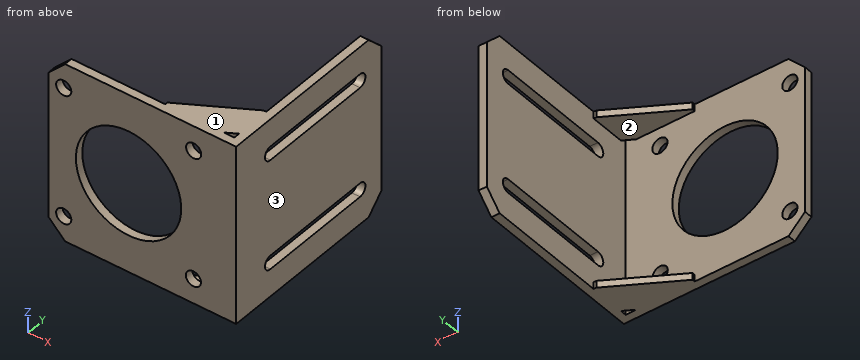
from build123d import *

# Parameters (mm, degrees)
SKETCH1_W           = 68
SKETCH1_H           = 65
BOSS_EXTRUDE1_DEPTH = 3
SKETCH2_W           = 3
SKETCH2_H           = 68
BOSS_EXTRUDE2_DEPTH = 65
CHAMFER1_SIZE       = 6
SKETCH4_R           = 2.75
SKETCH4_R_2         = 19.1
CUT_EXTRUDE2_DEPTH  = 65
CUT_EXTRUDE3_DEPTH  = 65
BOSS_EXTRUDE3_DEPTH = 2.5
BOSS_EXTRUDE4_DEPTH = 2.5


with BuildPart() as part:
    # Sketch1 → Boss-Extrude1 (new body)
    with BuildSketch(Plane(origin=(0, 0, 0), x_dir=(1, 0, 0), z_dir=(0, 1, 0))):
        Rectangle(SKETCH1_W, SKETCH1_H)
    extrude(amount=BOSS_EXTRUDE1_DEPTH)

    # Sketch2 → Boss-Extrude2 (add)
    with BuildSketch(Plane.XY.offset(32.5)):
        with Locations((32.5, 34)):
            Rectangle(SKETCH2_W, SKETCH2_H)
    extrude(amount=-BOSS_EXTRUDE2_DEPTH)

    # Chamfer1
    chamfer1_edges = [part.edges().sort_by_distance(p)[0] for p in [
        (32.5, 68, -32.5),
        (32.5, 68, 32.5),
        (-34, 1.5, -32.5),
        (-34, 1.5, 32.5),
    ]]
    chamfer(chamfer1_edges, length=CHAMFER1_SIZE)

    # Sketch4 → Cut-Extrude2 (cut)
    with BuildSketch(Plane(origin=(0, 3, 0), x_dir=(1, 0, 0), z_dir=(0, 1, 0))):
        with Locations(Location((-28.5, 23.5, 0), (0, 0, 270))):
            Circle(SKETCH4_R)
        with Locations(Location((-28.5, -23.5, 0), (0, 0, 270))):
            Circle(SKETCH4_R)
        with Locations(Location((18.6, -23.5, 0), (0, 0, 270))):
            Circle(SKETCH4_R)
        with Locations(Location((18.5, 23.5, 0), (0, 0, 270))):
            Circle(SKETCH4_R)
        with Locations(Location((-5, 0, 0), (0, 0, 270))):
            Circle(SKETCH4_R_2)
    extrude(amount=-CUT_EXTRUDE2_DEPTH, mode=Mode.SUBTRACT)

    # Sketch5 → Cut-Extrude3 (cut)
    with BuildSketch(Plane.ZY.offset(-31)):
        with BuildLine():
            Line((-17.5, 58), (-17.5, 16))
            ThreePointArc((-17.5, 16), (-20, 13.5), (-22.5, 16))
            Line((-22.5, 16), (-22.5, 58))
            ThreePointArc((-22.5, 58), (-20, 60.5), (-17.5, 58))
        make_face()
        with BuildLine():
            Line((22.5, 58), (22.5, 16))
            ThreePointArc((22.5, 16), (20, 13.5), (17.5, 16))
            Line((17.5, 16), (17.5, 58))
            ThreePointArc((17.5, 58), (20, 60.5), (22.5, 58))
        make_face()
    extrude(amount=-CUT_EXTRUDE3_DEPTH, mode=Mode.SUBTRACT)

    # Sketch6 → Boss-Extrude3 (add)
    with BuildSketch(Plane.XY.offset(32.5)):
        Polygon((6, 3), (6, 4), (30, 18), (31, 18), (31, 5.233358358), (27.171385671, 3), align=None)
    extrude(amount=-BOSS_EXTRUDE3_DEPTH)

    # Sketch7 → Boss-Extrude4 (add)
    with BuildSketch(Plane(origin=(0, 0, -32.5), x_dir=(-1, 0, 0), z_dir=(0, 0, -1))):
        Polygon((-31, 18), (-30, 18), (-6, 4), (-6, 3), (-27.171385671, 3), (-31, 5.233358358), align=None)
    extrude(amount=-BOSS_EXTRUDE4_DEPTH)


solid = part.part
Geometry: final body of the model. Coordinates: model frame, mm. Face numbers are marked on the shaded views. Give positions to 0.01 mm unless a question says otherwise; leave off trailing zeros. Loops run counter-clockwise (first coordinate to the right, second up) from the corner with the lowest first, then second, coordinate; pieces in that order, holes last. Notation, with made-up numbers: (5, 12) -> (28, 12) arc R17 ccw to (28, 24) -> close; hole circle Ø1 at (-19, 66.25). An arc over 180 degrees is marked (long way). Put each result on its own line as item: value.
1. Cut plane C-C (x = -16.5). Return the cut outline in (y, z), plus the area to 3 significant figures.
Taken from the geometry:
outline: (0, -32.5) -> (3, -32.5) -> (3, -15.25) -> (0, -15.25) -> close; (0, 15.25) -> (3, 15.25) -> (3, 32.5) -> (0, 32.5) -> close
area: 104 mm2
2. Pin query (flat end, axial travel): P1, Ø9, axis at x = 18.6, z = 23.5, coming from the +Y side; P2, Ø1.5, axis at y = 47.5, z = -9, coming from the -X side; P3, Ø0.8, axis at x = 30.5, z = -31, coming from the +Y side. Return the tip coordinate at first contact, or that it passes through.
Taken from the geometry:
P1: stops at y = 3
P2: stops at x = 31
P3: stops at y = 18
3. Cut plane D-D (z = 0). Return the cut outline in (x, y), plus the area to 3 significant figures.
Taken from the geometry:
outline: (-34, 0) -> (-24.1, 0) -> (-24.1, 3) -> (-34, 3) -> close; (14.1, 0) -> (34, 0) -> (34, 68) -> (31, 68) -> (31, 3) -> (14.1, 3) -> close
area: 284 mm2
4. Pull-direction query (Z, two-part tool) for the marked faces 1, 2 and 3; classes: released by +Z, released by -Z, zero draft, split by the parting line, or undercut.
Taken from the geometry:
face 1: released by +Z
face 2: undercut
face 3: zero draft
5. Cut plane A-A (y = 31). Return the cut outline in (x, z), plus the area to 3 significant figures.
Taken from the geometry:
outline: (31, -32.5) -> (34, -32.5) -> (34, -22.5) -> (31, -22.5) -> close; (31, -17.5) -> (34, -17.5) -> (34, 17.5) -> (31, 17.5) -> close; (31, 22.5) -> (34, 22.5) -> (34, 32.5) -> (31, 32.5) -> close
area: 165 mm2
6. Ray query, line 1 along X through (y, z) = (2, 0); line 2 along Z through (x, y) = (-28, 1); line 3 along Y through (x, z) = (8.5, -27). Return the intervals inside material, ascending. Write a range as [from, to].
Taken from the geometry:
line 1: x = [-34, -24.1], [14.1, 34]
line 2: z = [-32.5, -26.2], [-20.8, 20.8], [26.2, 32.5]
line 3: y = [0, 3]
7. Cut plane B-B (z = -23.5). Return the cut outline in (x, y).
Taken from the geometry:
outline: (-34, 0) -> (-31.25, 0) -> (-31.25, 3) -> (-34, 3) -> close; (-25.75, 0) -> (15.75, 0) -> (15.75, 3) -> (-25.75, 3) -> close; (21.25, 0) -> (34, 0) -> (34, 68) -> (31, 68) -> (31, 3) -> (21.25, 3) -> close
